Answer from the drawing. Dimensions are ordinates in mm from the lowest x, y and z of the part. A direction names the side the tool comes from. Give positions to 0.01 mm unless a question says otherwise; leave off trailing zeros. Write each loop counter-clockwise with the first axis right and the second up, starting at its lowest first coordinate (ties: lowest second). Pieces come first, ordered by that corner, then holes.
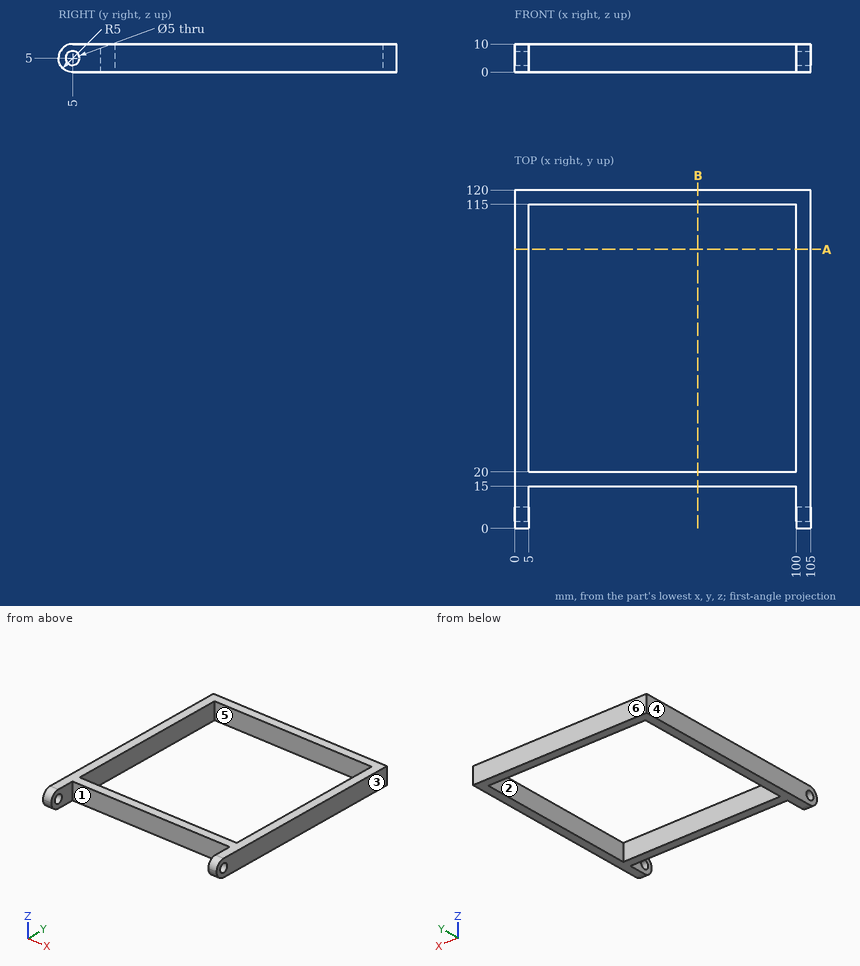
Item 1: A cutting plane is placed at B-B, the plane x = 65. Give the vertices of the cut face in (y, z), plus the area to 3 significant figures.
Conclusion:
outline: (15, 0) - (20, 0) - (20, 10) - (15, 10) - close; (115, 0) - (120, 0) - (120, 10) - (115, 10) - close
area: 100 mm2
Item 2: Each of these flat-tipped pins is pushed along its axis until it touches: P1, Ø3, axis at x = 48.5, z = 6, coming from the -Y side; P2, Ø3, axis at y = 5, z = 5, coming from the -X side. Where does it stop, or does it pass through?
Conclusion:
P1: stops at y = 15
P2: passes through
Item 3: Consider probe 1 along X at (y, z) = (68, 9); probe 2 along Y at (x, z) = (7, 3.25); probe 3 along Z at (x, y) = (103.5, 5). Determine where each line is inside the solid, lowest interval first.
Conclusion:
probe 1: x = 0 to 5, 100 to 105
probe 2: y = 15 to 20, 115 to 120
probe 3: z = 0 to 2.5, 7.5 to 10
Item 4: Determine the mould class of the marked faces 4, 5 and 6 for opening direction Y: pulls with the +Y half, pulls with the -Y half, needs draft (parallel to the pull), parting line crosses it, or undercut.
Conclusion:
face 4: needs draft
face 5: undercut
face 6: pulls with the +Y half
Item 5: Which of the six approach directions +Z, -Z, +X, -X, +Y, -Y give full straight-line access (tool end or side, diameter ignored) to the marked faces 1, 2 and 3?
Conclusion:
face 1: +Z, -Z, -Y
face 2: +Z, -Z
face 3: +Z, -Z, +X, +Y, -Y
Item 6: A cutting plane is placed at A-A, the plane y = 99. Give the vertices of the cut face in (x, z), plus the area to 3 significant figures.
Conclusion:
outline: (0, 0) - (5, 0) - (5, 10) - (0, 10) - close; (100, 0) - (105, 0) - (105, 10) - (100, 10) - close
area: 100 mm2
